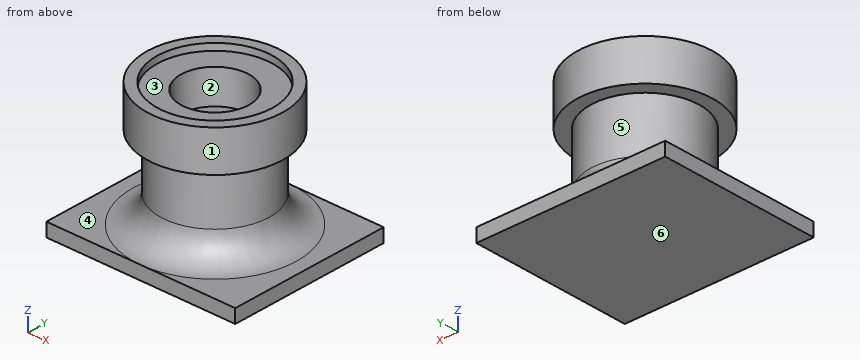
Autodesk Inventor part; units mm, degrees
ref_plane "YZ Plane" through (0, 0, 0) normal (1, 0, 0) x (0, 1, 0)
ref_plane "XZ Plane" through (0, 0, 0) normal (0, 1, 0) x (-1, 0, 0)
ref_plane "XY Plane" through (0, 0, 0) normal (0, 0, 1) x (1, 0, 0)
sketch "Sketch1" plane through (0, 0, 0) normal (0, 0, 1) x (1, 0, 0)
  line L0 (0, 0) -> (14, 0)
  line L1 (14, 0) -> (14, 12)
  line L2 (14, 12) -> (0, 12)
  line L3 (0, 12) -> (0, 0)
  dimension "d0" = 14
  dimension "d1" = 12
extrude "Extrusion1" add sketch "Sketch1" along normal blind 1
sketch "Sketch2" plane through (0, 0, 1) normal (0, 0, 1) x (1, 0, 0)
  line L0 (0, 0) -> (14, 0) construction
  line L1 (14, 0) -> (14, 12) construction
  line L2 (14, 12) -> (0, 12) construction
  line L3 (0, 12) -> (0, 0) construction
  circle A0 centre (7, 6) radius 4
  dimension "d4" = 8
extrude "Extrusion2" add sketch "Sketch2" along normal blind 6
sketch "Sketch3" plane through (7, 6, 7) normal (0, 0, 1) x (1, 0, 0)
  circle A0 centre (0, 0) radius 5
  circle A1 centre (0, 0) radius 3
  circle A2 centre (0, 0) radius 4
  point P0 (-7, -6)
  dimension "d7" = 10
  dimension "d8" = 6
extrude "Extrusion3" add sketch "Sketch3" along normal blind 3 contours A0 | A1 | A2
sketch "Sketch4" plane through (7, 6, 10) normal (0, 0, 1) x (1, 0, 0)
  circle A0 centre (0, 0) radius 2.5
  circle A1 centre (0, 0) radius 4.25
  circle A2 centre (0, 0) radius 5
  point P0 (-7, -6)
  dimension "d11" = 5
  dimension "d12" = 8.5
extrude "Extrusion4" cut sketch "Sketch4" against normal blind 3 contours A0
extrude "Extrusion5" cut sketch "Sketch4" against normal blind 0.5 contours A1
fillet "Fillet1" radius 2 1 edges at (3, 6, 1)
properties part number "Camera" material "ABS Plastic"
Verification items for the finished model (mm, model axes). Face numbers are marked on the shaded views. A direction names the side the tool comes from. Give positions to 0.01 mm unless a question says otherwise; leave off trailing zeros. Order: outer loops, then holes, each group sorted by start corner. A loop starts at its lowest first (then second) coordinate and runs counter-clockwise, first axis right, second up. Notation, with made-up numbers: M 84,13 L 106,13 A18 ccw 106,24 Z; hole C 32.5,14 d9. An arc over 180 degrees is marked long. Return JSON: item names as keys, results as strings. Group by question number.
1) Mould release check, pull along Y, two halves, no side actions. Record for the marked faces 1, 2, 3 and 4: pulls with the +Y half, pulls with the -Y half, needs draft (parallel to the pull), parting line crosses it, or undercut.
2) Scan lines: line 1 (Y direction, x = 7, z = 9.75); line 2 (Y direction, x = 7, z = 8.75); line 3 (Z direction, x = 2, y = 0.5). Record each from-to range of solid material in increasing order.
3) Section check D-D on z = 6. Record the cut outline in (x, y), and give its area (3 significant figures).
4) Access from +Z, -Z, +X, -X, +Y, -Y to the whole of each face (thin tool, end or side, straight path). Record for the marked faces 5 and 6.
5) Section check B-B on y = 6. Record the cut outline in (x, z), and give its area (3 significant figures).
6) Section check C-C on z = 9. Record the cut outline in (x, y).
7) Go/stop test with flat-tipped pins: pin 1 Ø5 at (y, z) = (10.5, 6.5) entering from -X; pin 2 Ø6 at (x, y) = (7, 6) entering from -Z; pin 3 Ø3 at (x, z) = (3, 4) entering from +Y; pin 4 Ø1.5 at (x, y) = (6, 5) entering from +Z. Record where each tip stops, or that it passes through.
Answer block:
{
 "1": {"face 1": "parting line crosses it", "face 2": "undercut", "face 3": "undercut", "face 4": "needs draft"},
 "2": {"line 1": "y = 1 to 1.75, 10.25 to 11", "line 2": "y = 1 to 3.5, 8.5 to 11", "line 3": "z = 0 to 1"},
 "3": {"outline": "C 7,6 d8", "area": "50.3 mm^2"},
 "4": {"face 5": "none", "face 6": "-Z, +X, -X, +Y, -Y"},
 "5": {"outline": "M 0,0 L 14,0 L 14,1 L 13,1 A2 cw 11,3 L 11,7 L 12,7 L 12,10 L 11.25,10 L 11.25,9.5 L 9.5,9.5 L 9.5,7 L 4.5,7 L 4.5,9.5 L 2.75,9.5 L 2.75,10 L 2,10 L 2,7 L 3,7 L 3,3 A2 cw 1,1 L 0,1 Z", "area": "77.0 mm^2"},
 "6": {"outline": "C 7,6 d10; hole C 7,6 d5"},
 "7": {"pin 1": "stops at x = 2.44", "pin 2": "stops at z = 0", "pin 3": "stops at y = 9.12", "pin 4": "stops at z = 7"}
}
